from build123d import *

# Parameters (mm, degrees)
SCHNITT_LINEAR_AUSTRAGEN1_DEPTH = 2
VERRUNDUNG1_R                   = 0.4
VERRUNDUNG2_R                   = 0.2


with BuildPart() as part:
    # Skizze1 → Rotation1 (revolve)
    with BuildSketch(Plane.XY):
        Polygon((0, 0), (0, -8), (-1, -8), (-1.5, -7.5), (-1.5, -3), (-2.7, -3), (-2.7, 0), align=None)
    revolve(axis=Axis((0, 0, 0), (0, -1, 0)))

    # Skizze2 → Schnitt-Linear austragen1 (cut)
    with BuildSketch(Plane(origin=(0, 0, 0), x_dir=(1, 0, 0), z_dir=(0, 1, 0))):
        Polygon((1.299038106, 0.75), (1.299038106, -0.75), (0, -1.5), (-1.299038106, -0.75), (-1.299038106, 0.75), (0, 1.5), align=None)
    extrude(amount=-SCHNITT_LINEAR_AUSTRAGEN1_DEPTH, mode=Mode.SUBTRACT)

    # Verrundung1
    verrundung1_edges = [part.edges().sort_by_distance(p)[0] for p in [
        (2.7, 0, 0),
        (2.7, -3, 0),
    ]]
    fillet(verrundung1_edges, radius=VERRUNDUNG1_R)

    # Verrundung2
    verrundung2_edges = [part.edges().sort_by_distance(p)[0] for p in [
        (0.649519053, 0, -1.125),
        (-0.649519053, 0, -1.125),
        (-1.299038106, 0, 0),
        (-0.649519053, 0, 1.125),
        (0.649519053, 0, 1.125),
        (1.299038106, 0, 0),
    ]]
    fillet(verrundung2_edges, radius=VERRUNDUNG2_R)


solid = part.part
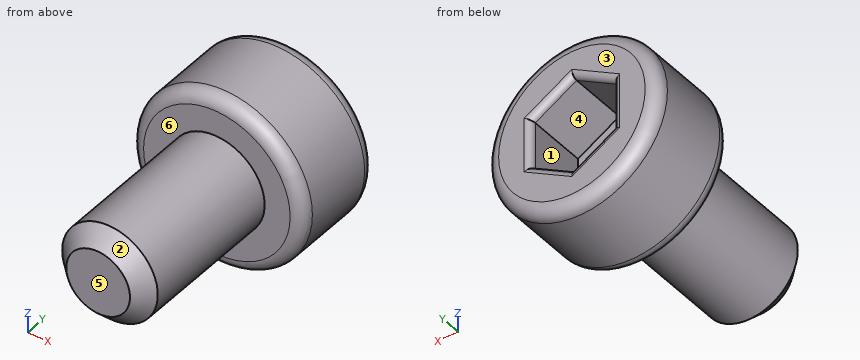
Verification items for the finished model (mm, model axes). Face numbers are marked on the shaded views. A direction names the side the tool comes from. Give positions to 0.01 mm unless a question says otherwise; leave off trailing zeros. Loops run counter-clockwise (first coordinate to the right, second up) from the corner with the lowest first, then second, coordinate; pieces in that order, holes last.
1) Sectioned sample at B-B, the plane y = -6.75. Enter the section's corners in (x, z), then the cut area to 3 significant figures.
2) Set-up check for the marked faces 4, 5 and 6: record each of +Z, -Z, +X, -X, +Y, -Y from which the full face is reachable in a straight line by a thin tool's end or side.
3) Depth check by flat-ended pin: pin 1 Ø1.5 at (x, y) = (0.5, -5) entering from +Z; pin 2 Ø1.5 at (x, y) = (-2, -1.5) entering from +Z; pin 3 Ø3 at (y, z) = (-1.5, 2) entering from +X. Enter the tip coordinate at first touch or a pass-through.
4) Draft check along Z on the marked faces 1, 2 and 3. Enter one of: pulls with the +Z half, pulls with the -Z half, needs draft (parallel to the pull), parting line crosses it, or undercut.
5) Sectioned sample at A-A, the plane z = 0. Enter the section's corners in (x, y).
6) Thickness scan on line 1 along Z through (x, y) = (1.3, -4.5); line 2 along X through (y, z) = (-1.25, -0.8); line 3 along Y through (x, z) = (-0.15, 1.7). Record the ranges inside material, lowest first.
Answers:
1. outline: circle Ø3 at (0, 0)
1. area: 7.07 mm2
2. face 4: +Y
2. face 5: +Z, -Z, +X, -X, -Y
2. face 6: -Y
3. pin 1: stops at z = 1.5
3. pin 2: stops at z = 2.39
3. pin 3: stops at x = 2.65
4. face 1: undercut
4. face 2: parting line crosses it
4. face 3: needs draft
5. outline: (-2.7, -2.6) arc R0.4 ccw to (-2.3, -3) - (-1.5, -3) - (-1.5, -7.5) - (-1, -8) - (1, -8) - (1.5, -7.5) - (1.5, -3) - (2.3, -3) arc R0.4 ccw to (2.7, -2.6) - (2.7, -0.4) arc R0.4 ccw to (2.3, 0) - (1.5, 0) arc R0.2 ccw to (1.3, -0.2) - (1.3, -2) - (-1.3, -2) - (-1.3, -0.2) arc R0.2 ccw to (-1.5, 0) - (-2.3, 0) arc R0.4 ccw to (-2.7, -0.4) - close
6. line 1: z = -0.75 to 0.75
6. line 2: x = -2.58 to -1.21, 1.21 to 2.58
6. line 3: y = -3 to 0
